Here's how the part is built. I have some questions about the finished solid (model axes, mm). Round coordinates to 2 decimals unless told otherwise and drop trailing zeros. Write each loop counter-clockwise with the first axis right and the second up, starting at its lowest first coordinate (ties: lowest second). Pieces come first, ordered by that corner, then holes. Notation, with made-up numbers: (3.25, -38.75) -> (28.25, -38.75) arc R24 ccw to (28.25, 0.25) -> close; hole circle Ø3 at (13.25, 88). An arc over 180 degrees is marked (long way). Answer in a Markdown table with one row per item.
from build123d import *

# Parameters (mm, degrees)
F0_R     = 10.5
F1_DEPTH = 1
F2_R     = 10.5
F3_DEPTH = 1


with BuildPart() as f1:
    # F0 (on Top) → F1 (new body)
    with BuildSketch(Plane.XY):
        with BuildLine():
            ThreePointArc((-114.9745469093, 28.0742291808), (-117.9034790975, 35.1452969927), (-124.9745469093, 38.0742291808))
            Line((-124.9745469093, 38.0742291808), (-216.9745469093, 38.0742291808))
            ThreePointArc((-216.9745469093, 38.0742291808), (-224.0456147212, 35.1452969927), (-226.9745469093, 28.0742291808))
            Line((-226.9745469093, 28.0742291808), (-226.9745469093, -63.9257708192))
            ThreePointArc((-226.9745469093, -63.9257708192), (-224.0456147212, -70.9968386311), (-216.9745469093, -73.9257708192))
            Line((-216.9745469093, -73.9257708192), (-124.9745469093, -73.9257708192))
            ThreePointArc((-124.9745469093, -73.9257708192), (-117.9034790975, -70.9968386311), (-114.9745469093, -63.9257708192))
            Line((-114.9745469093, -63.9257708192), (-114.9745469093, 28.0742291808))
        make_face()
        with Locations((-214.898198111, -61.8065597154)):
            Circle(F0_R, mode=Mode.SUBTRACT)
        with Locations((-192.898198111, -61.8065597154)):
            Circle(F0_R, mode=Mode.SUBTRACT)
        with Locations((-214.898198111, -39.8065597154)):
            Circle(F0_R, mode=Mode.SUBTRACT)
        with Locations((-192.898198111, -39.8065597154)):
            Circle(F0_R, mode=Mode.SUBTRACT)
        with Locations((-170.898198111, -61.8065597154)):
            Circle(F0_R, mode=Mode.SUBTRACT)
        with Locations((-148.898198111, -61.8065597154)):
            Circle(F0_R, mode=Mode.SUBTRACT)
        with Locations((-126.898198111, -61.8065597154)):
            Circle(F0_R, mode=Mode.SUBTRACT)
        with Locations((-170.898198111, -39.8065597154)):
            Circle(F0_R, mode=Mode.SUBTRACT)
        with Locations((-148.898198111, -39.8065597154)):
            Circle(F0_R, mode=Mode.SUBTRACT)
        with Locations((-126.898198111, -39.8065597154)):
            Circle(F0_R, mode=Mode.SUBTRACT)
        with Locations((-214.898198111, -17.8065597154)):
            Circle(F0_R, mode=Mode.SUBTRACT)
        with Locations((-214.898198111, 4.1934402846)):
            Circle(F0_R, mode=Mode.SUBTRACT)
        with Locations((-192.898198111, -17.8065597154)):
            Circle(F0_R, mode=Mode.SUBTRACT)
        with Locations((-192.898198111, 4.1934402846)):
            Circle(F0_R, mode=Mode.SUBTRACT)
        with Locations((-214.898198111, 26.1934402846)):
            Circle(F0_R, mode=Mode.SUBTRACT)
        with Locations((-192.898198111, 26.1934402846)):
            Circle(F0_R, mode=Mode.SUBTRACT)
        with Locations((-170.898198111, -17.8065597154)):
            Circle(F0_R, mode=Mode.SUBTRACT)
        with Locations((-148.898198111, -17.8065597154)):
            Circle(F0_R, mode=Mode.SUBTRACT)
        with Locations((-170.898198111, 4.1934402846)):
            Circle(F0_R, mode=Mode.SUBTRACT)
        with Locations((-148.898198111, 4.1934402846)):
            Circle(F0_R, mode=Mode.SUBTRACT)
        with Locations((-126.898198111, -17.8065597154)):
            Circle(F0_R, mode=Mode.SUBTRACT)
        with Locations((-126.898198111, 4.1934402846)):
            Circle(F0_R, mode=Mode.SUBTRACT)
        with Locations((-170.898198111, 26.1934402846)):
            Circle(F0_R, mode=Mode.SUBTRACT)
        with Locations((-148.898198111, 26.1934402846)):
            Circle(F0_R, mode=Mode.SUBTRACT)
        with Locations((-126.898198111, 26.1934402846)):
            Circle(F0_R, mode=Mode.SUBTRACT)
    extrude(amount=F1_DEPTH)

    # F2 (on face) → F3 (join)
    with BuildSketch(Plane.XY.offset(1)):
        with BuildLine():
            ThreePointArc((-114.9745469093, 28.0742291808), (-117.9034790975, 35.1452969927), (-124.9745469093, 38.0742291808))
            Line((-124.9745469093, 38.0742291808), (-216.9745469093, 38.0742291808))
            ThreePointArc((-216.9745469093, 38.0742291808), (-224.0456147212, 35.1452969927), (-226.9745469093, 28.0742291808))
            Line((-226.9745469093, 28.0742291808), (-226.9745469093, -63.9257708192))
            ThreePointArc((-226.9745469093, -63.9257708192), (-224.0456147212, -70.9968386311), (-216.9745469093, -73.9257708192))
            Line((-216.9745469093, -73.9257708192), (-124.9745469093, -73.9257708192))
            ThreePointArc((-124.9745469093, -73.9257708192), (-117.9034790975, -70.9968386311), (-114.9745469093, -63.9257708192))
            Line((-114.9745469093, -63.9257708192), (-114.9745469093, 28.0742291808))
        make_face()
        with Locations((-214.898198111, -61.8065597154)):
            Circle(F2_R, mode=Mode.SUBTRACT)
        with Locations((-192.898198111, -61.8065597154)):
            Circle(F2_R, mode=Mode.SUBTRACT)
        with Locations((-214.898198111, -39.8065597154)):
            Circle(F2_R, mode=Mode.SUBTRACT)
        with Locations((-192.898198111, -39.8065597154)):
            Circle(F2_R, mode=Mode.SUBTRACT)
        with Locations((-170.898198111, -61.8065597154)):
            Circle(F2_R, mode=Mode.SUBTRACT)
        with Locations((-148.898198111, -61.8065597154)):
            Circle(F2_R, mode=Mode.SUBTRACT)
        with Locations((-126.898198111, -61.8065597154)):
            Circle(F2_R, mode=Mode.SUBTRACT)
        with Locations((-170.898198111, -39.8065597154)):
            Circle(F2_R, mode=Mode.SUBTRACT)
        with Locations((-148.898198111, -39.8065597154)):
            Circle(F2_R, mode=Mode.SUBTRACT)
        with Locations((-126.898198111, -39.8065597154)):
            Circle(F2_R, mode=Mode.SUBTRACT)
        with Locations((-214.898198111, -17.8065597154)):
            Circle(F2_R, mode=Mode.SUBTRACT)
        with Locations((-214.898198111, 4.1934402846)):
            Circle(F2_R, mode=Mode.SUBTRACT)
        with Locations((-192.898198111, -17.8065597154)):
            Circle(F2_R, mode=Mode.SUBTRACT)
        with Locations((-192.898198111, 4.1934402846)):
            Circle(F2_R, mode=Mode.SUBTRACT)
        with Locations((-214.898198111, 26.1934402846)):
            Circle(F2_R, mode=Mode.SUBTRACT)
        with Locations((-192.898198111, 26.1934402846)):
            Circle(F2_R, mode=Mode.SUBTRACT)
        with Locations((-170.898198111, -17.8065597154)):
            Circle(F2_R, mode=Mode.SUBTRACT)
        with Locations((-148.898198111, -17.8065597154)):
            Circle(F2_R, mode=Mode.SUBTRACT)
        with Locations((-170.898198111, 4.1934402846)):
            Circle(F2_R, mode=Mode.SUBTRACT)
        with Locations((-148.898198111, 4.1934402846)):
            Circle(F2_R, mode=Mode.SUBTRACT)
        with Locations((-126.898198111, -17.8065597154)):
            Circle(F2_R, mode=Mode.SUBTRACT)
        with Locations((-126.898198111, 4.1934402846)):
            Circle(F2_R, mode=Mode.SUBTRACT)
        with Locations((-170.898198111, 26.1934402846)):
            Circle(F2_R, mode=Mode.SUBTRACT)
        with Locations((-148.898198111, 26.1934402846)):
            Circle(F2_R, mode=Mode.SUBTRACT)
        with Locations((-126.898198111, 26.1934402846)):
            Circle(F2_R, mode=Mode.SUBTRACT)
        with BuildLine():
            ThreePointArc((-114.9745469093, 28.0742291808), (-117.9034790975, 35.1452969927), (-124.9745469093, 38.0742291808))
            Line((-124.9745469093, 38.0742291808), (-216.9745469093, 38.0742291808))
            ThreePointArc((-216.9745469093, 38.0742291808), (-224.0456147212, 35.1452969927), (-226.9745469093, 28.0742291808))
            Line((-226.9745469093, 28.0742291808), (-226.9745469093, -63.9257708192))
            ThreePointArc((-226.9745469093, -63.9257708192), (-224.0456147212, -70.9968386311), (-216.9745469093, -73.9257708192))
            Line((-216.9745469093, -73.9257708192), (-124.9745469093, -73.9257708192))
            ThreePointArc((-124.9745469093, -73.9257708192), (-117.9034790975, -70.9968386311), (-114.9745469093, -63.9257708192))
            Line((-114.9745469093, -63.9257708192), (-114.9745469093, 28.0742291808))
        make_face()
    extrude(amount=F3_DEPTH)


solid = f1.part
1) I want a section at C-C, the plane y = 1. List the corners of the cut face in (x, z) for me.
Response:
| item | result |
|---|---|
| outline | (-226.97, 0) -> (-224.9, 0) -> (-224.9, 1) -> (-204.9, 1) -> (-204.9, 0) -> (-202.9, 0) -> (-202.9, 1) -> (-182.9, 1) -> (-182.9, 0) -> (-180.9, 0) -> (-180.9, 1) -> (-160.9, 1) -> (-160.9, 0) -> (-158.9, 0) -> (-158.9, 1) -> (-138.9, 1) -> (-138.9, 0) -> (-136.9, 0) -> (-136.9, 1) -> (-116.9, 1) -> (-116.9, 0) -> (-114.97, 0) -> (-114.97, 2) -> (-226.97, 2) -> close |
2) For pin 1 (12.5 mm diameter, centred on x = -214.9, y = -39.81, fed in from -Z), with a flat end and sliding along its axis, tell me the tip position at first contact or that it passes through.
Response:
| item | result |
|---|---|
| pin 1 | stops at z = 1 |
3) I want a section at A-A, the plane z = 0.45. Count the separate pieces of the cut face and the enclosed holes in it, and give its area (3 significant figures).
Response:
| item | result |
|---|---|
| separate pieces | 1 |
| enclosed holes | 25 |
| area | 3,800 mm^2 |
4) I want a section at B-B, the plane x = -169. List the corners of the cut face in (y, z) for me.
Response:
| item | result |
|---|---|
| outline | (-73.93, 0) -> (-72.13, 0) -> (-72.13, 1) -> (-51.48, 1) -> (-51.48, 0) -> (-50.13, 0) -> (-50.13, 1) -> (-29.48, 1) -> (-29.48, 0) -> (-28.13, 0) -> (-28.13, 1) -> (-7.48, 1) -> (-7.48, 0) -> (-6.13, 0) -> (-6.13, 1) -> (14.52, 1) -> (14.52, 0) -> (15.87, 0) -> (15.87, 1) -> (36.52, 1) -> (36.52, 0) -> (38.07, 0) -> (38.07, 2) -> (-73.93, 2) -> close |
5) I need wall thicknesses on line 1 (Y direction, x = -215, z = 0.6); line 2 (X direction, y = -3, z = 0.8); line 3 (X direction, y = 25, z = 0.5). Which ranges of each line are inside material? Lowest first, please. Write a range as [from, to].
Response:
| item | result |
|---|---|
| line 1 | y = [-73.93, -72.31], [-51.31, -50.31], [-29.31, -28.31], [-7.31, -6.31], [14.69, 15.69], [36.69, 38.07] |
| line 2 | x = [-226.97, -222.55], [-207.25, -200.55], [-185.25, -178.55], [-163.25, -156.55], [-141.25, -134.55], [-119.25, -114.97] |
| line 3 | x = [-226.97, -225.33], [-204.47, -203.33], [-182.47, -181.33], [-160.47, -159.33], [-138.47, -137.33], [-116.47, -114.97] |
6) We'd pull the mould along Y, two halves only. Please class faces 1 (the face through (-223.97, 35.22, 0.99)), 2 (the face through (-193, -40, 1)): +Y half, -Y half, draft (parallel to the pull), parting line (faces both ways), or undercut.
Response:
| item | result |
|---|---|
| face 1 | +Y half |
| face 2 | undercut |
